```python
from build123d import *

# Parameters (mm, degrees)
SKETCH1_W           = 87
SKETCH1_H           = 69.22
SKETCH1_R           = 2.125
BOSS_EXTRUDE1_DEPTH = 2
SKETCH2_R           = 4
SKETCH2_R_2         = 2.125
BOSS_EXTRUDE2_DEPTH = 7
SKETCH3_W           = 5.5
SKETCH3_H           = 23.5
CUT_EXTRUDE1_DEPTH  = 7
SKETCH4_R           = 2
CUT_EXTRUDE2_DEPTH  = 7
CUT_EXTRUDE3_DEPTH  = 5
SKETCH6_R           = 2
CUT_EXTRUDE4_DEPTH  = 10
FILLET1_R           = 1
FILLET2_R           = 2.54


with BuildPart() as part:
    # Sketch1 → Boss-Extrude1 (new body)
    with BuildSketch(Plane(origin=(0, 0, 0), x_dir=(1, 0, 0), z_dir=(0, 1, 0))):
        Rectangle(SKETCH1_W, SKETCH1_H)
        with Locations((-38.1, 29.21)):
            Circle(SKETCH1_R, mode=Mode.SUBTRACT)
        with Locations((38.1, 29.21)):
            Circle(SKETCH1_R, mode=Mode.SUBTRACT)
        with Locations((-20.32, 29.21)):
            Circle(SKETCH1_R, mode=Mode.SUBTRACT)
        with Locations((38.1, -29.21)):
            Circle(SKETCH1_R, mode=Mode.SUBTRACT)
    extrude(amount=BOSS_EXTRUDE1_DEPTH)

    # Sketch2 → Boss-Extrude2 (add)
    with BuildSketch(Plane.XZ):
        with Locations((38.1, -29.21)):
            Circle(SKETCH2_R)
        with Locations((38.1, -29.21)):
            Circle(SKETCH2_R_2, mode=Mode.SUBTRACT)
        with Locations((-20.32, -29.21)):
            Circle(SKETCH2_R)
        with Locations((-20.32, -29.21)):
            Circle(SKETCH2_R_2, mode=Mode.SUBTRACT)
        with Locations((-38.1, -29.21)):
            Circle(SKETCH2_R)
        with Locations((-38.1, -29.21)):
            Circle(SKETCH2_R_2, mode=Mode.SUBTRACT)
        with Locations((38.1, 29.21)):
            Circle(SKETCH2_R)
        with Locations((38.1, 29.21)):
            Circle(SKETCH2_R_2, mode=Mode.SUBTRACT)
    extrude(amount=BOSS_EXTRUDE2_DEPTH)

    # Sketch3 → Cut-Extrude1 (cut)
    with BuildSketch(Plane(origin=(0, 2, 0), x_dir=(1, 0, 0), z_dir=(0, 1, 0))):
        with Locations((-40.75, 11.36)):
            Rectangle(SKETCH3_W, SKETCH3_H)
    extrude(amount=-CUT_EXTRUDE1_DEPTH, mode=Mode.SUBTRACT)

    # Sketch4 → Cut-Extrude2 (cut)
    with BuildSketch(Plane(origin=(0, 2, 0), x_dir=(1, 0, 0), z_dir=(0, 1, 0))):
        with Locations((-38.59, -28.97)):
            Circle(SKETCH4_R)
        with Locations((-38.59, -18.81)):
            Circle(SKETCH4_R)
        with Locations((-35.3, 10.16)):
            Circle(SKETCH4_R)
    extrude(amount=-CUT_EXTRUDE2_DEPTH, mode=Mode.SUBTRACT)

    # Sketch5 → Cut-Extrude3 (cut)
    with BuildSketch(Plane(origin=(0, 2, 0), x_dir=(1, 0, 0), z_dir=(0, 1, 0))):
        with BuildLine():
            Line((-23.732050808, 19.61), (-21.422649731, 23.61))
            ThreePointArc((-21.422649731, 23.61), (-18.690598923, 24.342050808), (-17.958548116, 21.61))
            Line((-17.958548116, 21.61), (-20.267949192, 17.61))
            ThreePointArc((-20.267949192, 17.61), (-23, 16.877949192), (-23.732050808, 19.61))
        make_face()
        with BuildLine():
            Line((-23.732050808, 3.557422926), (-12.154690036, 23.61))
            ThreePointArc((-12.154690036, 23.61), (-9.422639229, 24.342050808), (-8.690588421, 21.61))
            Line((-8.690588421, 21.61), (-20.267949192, 1.557422926))
            ThreePointArc((-20.267949192, 1.557422926), (-23, 0.825372119), (-23.732050808, 3.557422926))
        make_face()
        with BuildLine():
            Line((-23.732050808, -12.495154147), (-2.886730341, 23.61))
            ThreePointArc((-2.886730341, 23.61), (-0.154679534, 24.342050808), (0.577371274, 21.61))
            Line((0.577371274, 21.61), (-20.267949192, -14.495154147))
            ThreePointArc((-20.267949192, -14.495154147), (-23, -15.227204955), (-23.732050808, -12.495154147))
        make_face()
        with BuildLine():
            Line((9.845330968, 21.61), (-17.417148743, -25.61))
            ThreePointArc((-17.417148743, -25.61), (-20.14919955, -26.342050808), (-20.881250358, -23.61))
            Line((-20.881250358, -23.61), (6.381229353, 23.61))
            ThreePointArc((6.381229353, 23.61), (9.113280161, 24.342050808), (9.845330968, 21.61))
        make_face()
        with BuildLine():
            Line((-11.613290663, -23.61), (15.649189048, 23.61))
            ThreePointArc((15.649189048, 23.61), (18.381239856, 24.342050808), (19.113290663, 21.61))
            Line((19.113290663, 21.61), (-8.149189048, -25.61))
            ThreePointArc((-8.149189048, -25.61), (-10.881239856, -26.342050808), (-11.613290663, -23.61))
        make_face()
        with BuildLine():
            Line((28.381250358, 21.61), (1.118770647, -25.61))
            ThreePointArc((1.118770647, -25.61), (-1.613280161, -26.342050808), (-2.345330968, -23.61))
            Line((-2.345330968, -23.61), (24.917148743, 23.61))
            ThreePointArc((24.917148743, 23.61), (27.64919955, 24.342050808), (28.381250358, 21.61))
        make_face()
        with BuildLine():
            Line((6.922628726, -23.61), (27.767949192, 12.495154147))
            ThreePointArc((27.767949192, 12.495154147), (30.5, 13.227204955), (31.232050808, 10.495154147))
            Line((31.232050808, 10.495154147), (10.386730341, -25.61))
            ThreePointArc((10.386730341, -25.61), (7.654679534, -26.342050808), (6.922628726, -23.61))
        make_face()
        with BuildLine():
            Line((31.232050808, -5.557422926), (19.654690036, -25.61))
            ThreePointArc((19.654690036, -25.61), (16.922639229, -26.342050808), (16.190588421, -23.61))
            Line((16.190588421, -23.61), (27.767949192, -3.557422926))
            ThreePointArc((27.767949192, -3.557422926), (30.5, -2.825372119), (31.232050808, -5.557422926))
        make_face()
        with BuildLine():
            Line((25.458548116, -23.61), (27.767949192, -19.61))
            ThreePointArc((27.767949192, -19.61), (30.5, -18.877949192), (31.232050808, -21.61))
            Line((31.232050808, -21.61), (28.922649731, -25.61))
            ThreePointArc((28.922649731, -25.61), (26.190598923, -26.342050808), (25.458548116, -23.61))
        make_face()
    extrude(amount=-CUT_EXTRUDE3_DEPTH, mode=Mode.SUBTRACT)

    # Sketch6 → Cut-Extrude4 (cut)
    with BuildSketch(Plane(origin=(0, 2, 0), x_dir=(1, 0, 0), z_dir=(0, 1, 0))):
        with Locations((-30.2, 2.54)):
            Circle(SKETCH6_R)
    extrude(amount=-CUT_EXTRUDE4_DEPTH, mode=Mode.SUBTRACT)

    # Fillet1
    fillet1_edges = [part.edges().sort_by_distance(p)[0] for p in [
        (-38, 1, -23.11),
        (-38, 1, 0.39),
        (-43.5, 1, 0.39),
        (-43.5, 1, -23.11),
    ]]
    fillet(fillet1_edges, radius=FILLET1_R)

    # Fillet2
    fillet2_edges = [part.edges().sort_by_distance(p)[0] for p in [
        (-43.5, 1, 34.61),
        (-43.5, 1, -34.61),
        (43.5, 1, -34.61),
        (43.5, 1, 34.61),
    ]]
    fillet(fillet2_edges, radius=FILLET2_R)


solid = part.part
```
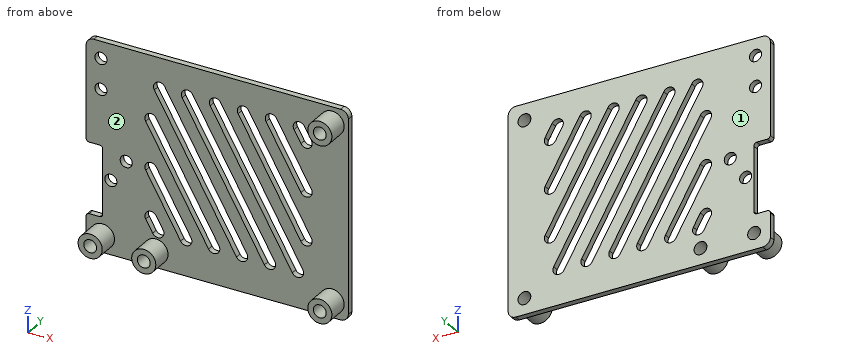
Here's how the part is built. I have some questions about the finished solid (model axes, mm). Face numbers are marked on the shaded views. Give positions to 0.01 mm unless a question says otherwise; leave off trailing zeros. Order: outer loops, then holes, each group sorted by start corner. A loop starts at its lowest first (then second) coordinate and runs counter-clockwise, first axis right, second up. Notation, with made-up numbers: M -33,40.25 L 19,40.25 A28 ccw 19,72.25 Z; hole C 24.5,84.5 d8. An arc over 180 degrees is marked long. Use a Markdown table: item, result. Add a question column.
1. Suppose I cut it at C-C (z = -14.5). List the corners of the cut face in (x, y) for me, and give its area (3 significant figures).
2. If we mould it in two halves opening along X, with no side actions, what happens to the marked faces 1 and 2? For each: +X half, -X half, draft (parallel to the pull), parting line (faces both ways), or undercut.
3. Suppose I cut it at B-B (x = 38.1). List the corners of the cut face in (y, z) for me (3 decimals).
4. For pin 1 Ø1 at (y, z) = (1, -12.5) entering from -X; pin 2 Ø2.5 at (x, z) = (38.1, -29.21) entering from -Y; pin 3 Ø3 at (x, y) = (-33.5, -4.5) entering from +Z; pin 4 Ø5 at (x, z) = (-35.3, -10.16) entering from -Y, each with a flat end and sliding along its axis, tell me the tip position at first contact or that it passes through.
5. I need wall thicknesses on probe 1 along Z at (x, y) = (-38.1, -4.75) (3 decimals); probe 2 along Y at (x, z) = (-25.5, -3.5); probe 3 along X at (y, z) = (-3.25, 29). Which ranges of each line are inside material? Lowest first, please. Write a range as from..to.
6. Suppose I cut it at D-D (x = -30). List the corners of the cut face in (y, z) for me, and give its area (3 significant figures).
7. Suppose I cut it at A-A (y = -5.25). List the corners of the cut face in (x, z) for me (3 decimals), and give its area (3 significant figures).
Results list:
| question | item | result |
|---|---|---|
| 1 | outline | M -38,0 L -17.41,0 L -17.41,2 L -38,2 Z; M -12.8,0 L -8.15,0 L -8.15,2 L -12.8,2 Z; M -3.53,0 L 1.12,0 L 1.12,2 L -3.53,2 Z; M 5.74,0 L 10.39,0 L 10.39,2 L 5.74,2 Z; M 15.01,0 L 19.66,0 L 19.66,2 L 15.01,2 Z; M 24.28,0 L 43.5,0 L 43.5,2 L 24.28,2 Z |
| 1 | area | 117 mm² |
| 2 | face 1 | draft |
| 2 | face 2 | undercut |
| 3 | outline | M -7,-33.21 L 0,-33.21 L 0,-34.61 L 2,-34.61 L 2,-31.335 L -7,-31.335 Z; M -7,-27.085 L 2,-27.085 L 2,27.085 L -7,27.085 L -7,25.21 L 0,25.21 L 0,-25.21 L -7,-25.21 Z; M -7,31.335 L 2,31.335 L 2,34.61 L 0,34.61 L 0,33.21 L -7,33.21 Z |
| 4 | pin 1 | stops at x = -38 |
| 4 | pin 2 | passes through |
| 4 | pin 3 | stops at z = -26.68 |
| 4 | pin 4 | stops at y = 0 |
| 5 | probe 1 | z = -33.21..-31.335, -27.085..-25.21 |
| 5 | probe 2 | y = 0..2 |
| 5 | probe 3 | x = 34.11..35.99, 40.21..42.09 |
| 6 | outline | M 0,-34.61 L 2,-34.61 L 2,-4.53 L 0,-4.53 Z; M 0,-0.55 L 2,-0.55 L 2,34.61 L 0,34.61 Z |
| 6 | area | 130 mm² |
| 7 | outline | C -38.1,-29.21 d8; C -20.32,-29.21 d8; C 38.1,-29.21 d8; C 38.1,29.21 d8; hole C -38.1,-29.21 d4.25; hole C -20.32,-29.21 d4.25; hole C 38.1,-29.21 d4.25; hole C 38.1,29.21 d4.25 |
| 7 | area | 144 mm² |
